from build123d import *

# Parameters (mm, degrees)
BOSS_EXTRUDE2_DEPTH  = 123
CUT_EXTRUDE2_DEPTH   = 118
SKETCH4_W            = 236
SKETCH4_H            = 60.975887641
CUT_EXTRUDE3_DEPTH   = 2.5
CUT_EXTRUDE4_DEPTH   = 2.5
BOSS_EXTRUDE4_DEPTH  = 10
SKETCH15_W           = 10
SKETCH15_H           = 10
SKETCH15_W_2         = 9
SKETCH15_H_2         = 9
SKETCH15_W_3         = 10.002299771
SKETCH15_W_4         = 9.002299771
BOSS_EXTRUDE14_DEPTH = 10


with BuildPart() as part:
    # Sketch1 → Boss-Extrude2 (new, symmetric)
    with BuildSketch(Plane(origin=(0, 0, 0), x_dir=(0, 0, -1), z_dir=(1, 0, 0))):
        Polygon((42.073890907, 65.041424054), (127.810405881, 15.541424054), (127.810405881, -14.715701058), (-3.083986323, -14.715701058), (-3.083986323, 10.284298942), align=None)
    extrude(amount=BOSS_EXTRUDE2_DEPTH, both=True)

    # Sketch3 → Cut-Extrude2 (cut, symmetric)
    with BuildSketch(Plane(origin=(0, 0, 0), x_dir=(0, 0, -1), z_dir=(1, 0, 0))):
        Polygon((43.238822658, 58.595347702), (1.916013677, 8.488514516), (1.916013677, -9.715701058), (122.810405881, -9.715701058), (122.810405881, 12.654672708), align=None)
    extrude(amount=CUT_EXTRUDE2_DEPTH, both=True, mode=Mode.SUBTRACT)

    # Sketch4 → Cut-Extrude3 (cut)
    with BuildSketch(Plane(origin=(0, 5.676918447, 6.883665768), x_dir=(1, 0, 0), z_dir=(0, 0.6362425146167643, 0.7714891202046446))):
        with Locations((0, 41.460005351)):
            Rectangle(SKETCH4_W, SKETCH4_H)
    extrude(amount=-CUT_EXTRUDE3_DEPTH, mode=Mode.SUBTRACT)

    # Sketch5 → Cut-Extrude4 (cut)
    with BuildSketch(Plane(origin=(0, 4.08631216, 4.954942968), x_dir=(1, 0, 0), z_dir=(0, 0.6362425146167643, 0.7714891202046446))):
        Polygon((107.577700229, 69.447949171), (107.997700229, 69.447949171), (107.997700229, 62.714644326), (115.5, 62.714644326), (115.5, 62.664644326), (115.5, 62.614644326), (115.5, 62.447949171), (115.5, 20.47206153), (107.997700229, 20.47206153), (107.997700229, 13.47206153), (-107.997700229, 13.47206153), (-107.997700229, 20.47206153), (-115.5, 20.47206153), (-115.5, 62.714644326), (-107.997700229, 62.714644326), (-107.997700229, 69.447949171), align=None)
    extrude(amount=-CUT_EXTRUDE4_DEPTH, mode=Mode.SUBTRACT)

    # Sketch6 → Boss-Extrude4 (add)
    with BuildSketch(Plane.ZY.offset(123)):
        Polygon((-73.692184958, 7.957950111), (-98.764682853, 20.186624411), (-44.520247585, 51.504663714), (-19.185344447, 20.784298942), (-78.102547156, 20.784298942), (-34.801276967, -4.215701058), (-126.884199241, -4.215701058), align=None)
    boss_extrude4 = extrude(amount=BOSS_EXTRUDE4_DEPTH)

    # Mirror1: Boss-Extrude4 across plane
    add(boss_extrude4.mirror(Plane(origin=(0, 0, 0), x_dir=(0, 0, 1), z_dir=(1, 0, 0))))

    # Sketch15 → Boss-Extrude14 (add)
    # profile 1 of 4: a face of its own
    with BuildSketch(Plane(origin=(0, 2.495705874, 3.026220167), x_dir=(-1, 0, 0), z_dir=(0, -0.6362425146167643, -0.7714891202046446))):
        with Locations((-113, 67.716050504)):
            Rectangle(SKETCH15_W, SKETCH15_H)
        with Locations((-113, 67.716050504)):
            Rectangle(SKETCH15_W_2, SKETCH15_H_2, mode=Mode.SUBTRACT)
    # profile 2 of 4: a face of its own
    with BuildSketch(Plane(origin=(0, 2.495705874, 3.026220167), x_dir=(-1, 0, 0), z_dir=(0, -0.6362425146167643, -0.7714891202046446))):
        with Locations((113, 67.716050504)):
            Rectangle(SKETCH15_W, SKETCH15_H)
        with Locations((113, 67.716050504)):
            Rectangle(SKETCH15_W_2, SKETCH15_H_2, mode=Mode.SUBTRACT)
    # profile 3 of 4: a face of its own
    with BuildSketch(Plane(origin=(0, 2.495705874, 3.026220167), x_dir=(-1, 0, 0), z_dir=(0, -0.6362425146167643, -0.7714891202046446))):
        with Locations((-112.998850115, 15.47206153)):
            Rectangle(SKETCH15_W_3, SKETCH15_H)
        with Locations((-112.998850115, 15.47206153)):
            Rectangle(SKETCH15_W_4, SKETCH15_H_2, mode=Mode.SUBTRACT)
    # profile 4 of 4: a face of its own
    with BuildSketch(Plane(origin=(0, 2.495705874, 3.026220167), x_dir=(-1, 0, 0), z_dir=(0, -0.6362425146167643, -0.7714891202046446))):
        with Locations((112.998850115, 15.47206153)):
            Rectangle(SKETCH15_W_3, SKETCH15_H)
        with Locations((112.998850115, 15.47206153)):
            Rectangle(SKETCH15_W_4, SKETCH15_H_2, mode=Mode.SUBTRACT)
    extrude(amount=BOSS_EXTRUDE14_DEPTH)


solid = part.part
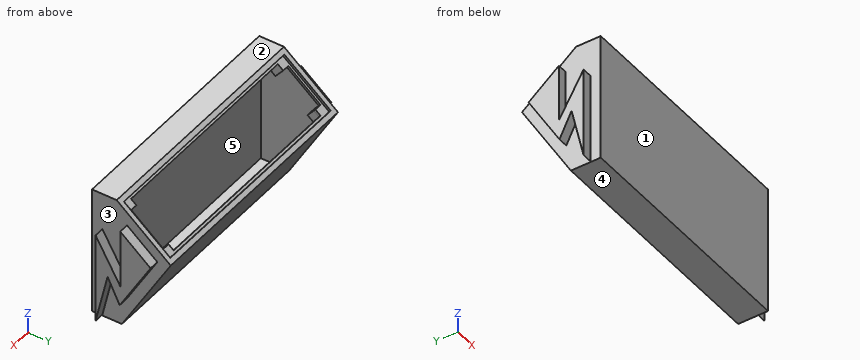
Read the model definition and answer for the solid it produces. Units are mm, in the model's axes. Face numbers are marked on the shaded views. A direction names the side the tool comes from. Round coordinates to 2 decimals unless told otherwise and drop trailing zeros. Write each loop counter-clockwise with the first axis right and the second up, starting at its lowest first coordinate (ties: lowest second). Pieces come first, ordered by that corner, then holes.
Q1. Straight lines are drawn through the part: line 1 (Z direction, x = -115, y = -3); line 2 (X direction, y = 3.5, z = -84); line 3 (X direction, y = 13, z = -63.5). For each, find the intervals that lie inside material, in ascending order.
Values:
line 1: z = -127.81 to -122.81, -1.92 to 3.08
line 2: x = -133 to -118, 118 to 133
line 3: x = -123 to -118, 118 to 123
Q2. Find section C-C on x = 52.5. Determine the outline of the cut face in (y, z), and give its area (3 significant figures).
Values:
outline: (-14.72, -127.81) - (15.54, -127.81) - (65.04, -42.07) - (61.18, -38.89) - (59.59, -40.82) - (57.66, -39.23) - (56.07, -41.16) - (58.6, -43.24) - (12.65, -122.81) - (-9.72, -122.81) - (-9.72, -1.92) - (8.49, -1.92) - (12.89, -5.55) - (14.48, -3.62) - (12.55, -2.03) - (14.14, -0.1) - (10.28, 3.08) - (-14.72, 3.08) - close
area: 1,390 mm2
Q3. A tool of negligible diameter and unlimited length cuts with its end or side. For the marked faces 4 and 5, from which of +Z, -Z, +X, -X, +Y, -Y can it reach the whole face along a straight path? Write none if from no direction.
Values:
face 4: -Z, +X, -X, +Y, -Y
face 5: none
Q4. Find section D-D on z = -112.5. Determine the outline of the cut face in (x, y).
Values:
outline: (-133, -4.22) - (-123, -4.22) - (-123, -14.72) - (123, -14.72) - (123, -4.22) - (133, -4.22) - (133, -0.92) - (123, -0.92) - (123, 24.38) - (-123, 24.38) - (-123, -0.92) - (-133, -0.92) - close; hole (-118, -9.72) - (118, -9.72) - (118, 18.61) - (-118, 18.61) - close
Q5. Find section A-A on z = -63. Determine the outline of the cut face in (x, y), and give its area (3 significant figures).
Values:
outline: (-133, -4.22) - (-123, -4.22) - (-123, -14.72) - (123, -14.72) - (123, -4.22) - (133, -4.22) - (133, 12.06) - (123, 12.06) - (123, 20.78) - (133, 20.78) - (133, 40.84) - (123, 40.84) - (123, 52.96) - (-123, 52.96) - (-123, 40.84) - (-133, 40.84) - (-133, 20.78) - (-123, 20.78) - (-123, 12.06) - (-133, 12.06) - close; hole (-118, -9.72) - (118, -9.72) - (118, 47.19) - (-118, 47.19) - close
area: 3,950 mm2
Q6. Flat-ended cylindrical pins translate along their axes: P1, Ø7, axis at y = 8.5, z = -12.5, coming from the +X side; P2, Ø10, axis at x = 41, y = 36, coming from the -Z side; P3, Ø6, axis at y = 30.5, z = -111.5, coming from the -X side; P4, Ø2, axis at y = 32, z = -100, coming from the -X side. Find the tip coordinate at first contact, or state that the pin passes through.
Values:
P1: stops at x = 123
P2: stops at z = -101.04
P3: passes through
P4: stops at x = -123
Q7. The mould has two halves that part along Y. Classify the marked faces 1, 2 and 3: released by +Y, released by -Y, zero draft, split by the parting line, or undercut.
Values:
face 1: released by -Y
face 2: zero draft
face 3: undercut
Q8. Find section B-B on y = 25. Determine the outline of the cut face in (x, z), and give its area (3 significant figures).
Values:
outline: (-133, -90.43) - (-123, -90.43) - (-123, -111.43) - (123, -111.43) - (123, -90.43) - (133, -90.43) - (133, -22.66) - (123, -22.66) - (123, -9.05) - (118, -9.05) - (118, -12.29) - (115.5, -12.29) - (115.5, -15.53) - (118, -15.53) - (118, -101.43) - (-118, -101.43) - (-118, -15.53) - (-115.5, -15.53) - (-115.5, -12.29) - (-118, -12.29) - (-118, -9.05) - (-123, -9.05) - (-123, -22.66) - (-133, -22.66) - close
area: 4,760 mm2
